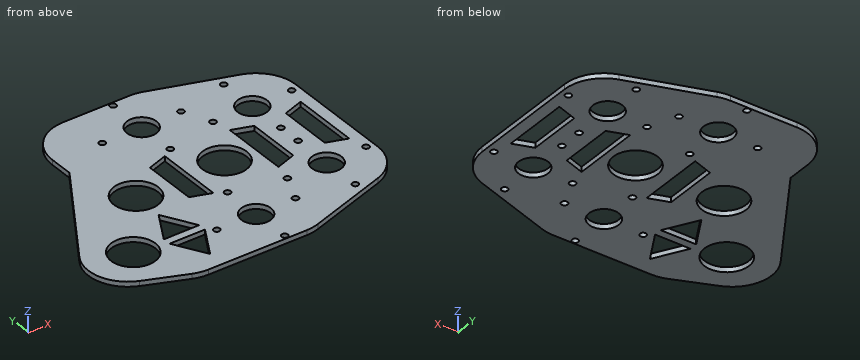
```python
from build123d import *

# Parameters (mm, degrees)
SKETCH1_R           = 14.2875
SKETCH1_R_2         = 9.525
BASE_FLANGE1_DEPTH  = 3.175
SKETCH2_R           = 2.032
CUT_EXTRUDE1_DEPTH  = 3.175
BREAK_CORNER1_START = -3.175
BREAK_CORNER1_DEPTH = 3.175
CUT_EXTRUDE2_DEPTH  = 3.175


# Read off the part's stored shape, not the designer's step: Break-Corner1
# Sheet-metal steps are written as plain solids
with BuildPart() as part:
    # Sketch1 → Base-Flange1 (new body)
    with BuildSketch(Plane.XY):
        Polygon((-72.39, 38.1), (-72.39, 78.74), (0, 78.74), (72.39, 54.946557626), (72.39, -54.946557626), (0, -78.74), (-72.39, -78.74), (-131.261342758, -54.940525177), align=None)
        Circle(SKETCH1_R, mode=Mode.SUBTRACT)
        with Locations((-16.51, 50.800692145)):
            Circle(SKETCH1_R_2, mode=Mode.SUBTRACT)
        with Locations(Location((-16.51, -50.800692145, 0), (0, 0, 180))):
            Circle(SKETCH1_R_2, mode=Mode.SUBTRACT)
        with Locations((-57.15, 0)):
            Circle(SKETCH1_R, mode=Mode.SUBTRACT)
        with Locations((-89.654815243, -42.291755533)):
            Circle(SKETCH1_R, mode=Mode.SUBTRACT)
        with Locations((41.987736572, 33.02)):
            Circle(SKETCH1_R_2, mode=Mode.SUBTRACT)
        with Locations((41.987736572, -33.02)):
            Circle(SKETCH1_R_2, mode=Mode.SUBTRACT)
    extrude(amount=-BASE_FLANGE1_DEPTH)

    # Sketch2 → Cut-Extrude1 (cut)
    with BuildSketch(Plane.XY):
        with Locations((-16.51, 76.200692145)):
            Circle(SKETCH2_R)
        with Locations((8.89, 50.800692145)):
            Circle(SKETCH2_R)
        with Locations(Location((-16.51, 25.400692145, 0), (0, 0, 180))):
            Circle(SKETCH2_R)
        with Locations(Location((-41.91, 50.800692145, 0), (0, 0, 180))):
            Circle(SKETCH2_R)
        with Locations((-41.91, -50.800692145)):
            Circle(SKETCH2_R)
        with Locations(Location((-16.51, -76.200692145, 0), (0, 0, 180))):
            Circle(SKETCH2_R)
        with Locations(Location((8.89, -50.800692145, 0), (0, 0, 180))):
            Circle(SKETCH2_R)
        with Locations((-16.51, -25.400692145)):
            Circle(SKETCH2_R)
        with Locations((41.987736572, 58.42)):
            Circle(SKETCH2_R)
        with Locations(Location((41.987736572, 7.62, 0), (0, 0, 180))):
            Circle(SKETCH2_R)
        with Locations((16.587736572, 33.02)):
            Circle(SKETCH2_R)
        with Locations(Location((67.387736572, 33.02, 0), (0, 0, 180))):
            Circle(SKETCH2_R)
        with Locations((41.987736572, -7.62)):
            Circle(SKETCH2_R)
        with Locations((67.387736572, -33.02)):
            Circle(SKETCH2_R)
        with Locations(Location((41.987736572, -58.42, 0), (0, 0, 180))):
            Circle(SKETCH2_R)
        with Locations(Location((16.587736572, -33.02, 0), (0, 0, 180))):
            Circle(SKETCH2_R)
    extrude(amount=-CUT_EXTRUDE1_DEPTH, mode=Mode.SUBTRACT)

    # Break-Corner1 outline → Break-Corner1 (cut)
    with BuildSketch(Plane.XY.offset(BREAK_CORNER1_START)):
        with BuildLine():
            ThreePointArc((-72.39, 53.34), (-64.950512242, 71.300512242), (-46.99, 78.74))
            Line((-46.99, 78.74), (-72.39, 78.74))
            Line((-72.39, 78.74), (-72.39, 53.34))
        make_face()
        with BuildLine():
            Line((0, 78.74), (-4.067255107, 78.74))
            ThreePointArc((-4.067255107, 78.74), (-0.051162479, 78.420490426), (3.863892351, 77.47))
            Line((3.863892351, 77.47), (0, 78.74))
        make_face()
        with BuildLine():
            ThreePointArc((-103.041642579, -66.34869106), (-117.701544329, -50.578489915), (-114.985920109, -29.218776702))
            Line((-114.985920109, -29.218776702), (-131.261342758, -54.940525177))
            Line((-131.261342758, -54.940525177), (-103.041642579, -66.34869106))
        make_face()
        with BuildLine():
            Line((72.39, 54.946557626), (54.921147458, 60.688291792))
            ThreePointArc((54.921147458, 60.688291792), (67.564391187, 51.453070316), (72.39, 36.558291792))
            Line((72.39, 36.558291792), (72.39, 54.946557626))
        make_face()
        with BuildLine():
            ThreePointArc((-67.450063518, -78.74), (-72.299143718, -78.27283821), (-76.969853447, -76.888537103))
            Line((-76.969853447, -76.888537103), (-72.39, -78.74))
            Line((-72.39, -78.74), (-67.450063518, -78.74))
        make_face()
        with BuildLine():
            Line((72.39, -54.946557626), (72.39, -36.558291792))
            ThreePointArc((72.39, -36.558291792), (67.564391187, -51.453070316), (54.921147458, -60.688291792))
            Line((54.921147458, -60.688291792), (72.39, -54.946557626))
        make_face()
        with BuildLine():
            ThreePointArc((3.863892351, -77.47), (-0.051162479, -78.420490426), (-4.067255107, -78.74))
            Line((-4.067255107, -78.74), (0, -78.74))
            Line((0, -78.74), (3.863892351, -77.47))
        make_face()
    extrude(amount=BREAK_CORNER1_DEPTH, mode=Mode.SUBTRACT)

    # Sketch3 → Cut-Extrude2 (cut)
    with BuildSketch(Plane.XY):
        Polygon((64.847736572, 21.59), (64.847736572, -21.59), (52.147736572, -17.272), (52.147736572, 17.272), align=None)
        Polygon((19.127736572, 21.59), (19.127736572, -21.59), (31.827736572, -17.272), (31.827736572, 17.272), align=None)
        Polygon((-35.56, -17.272), (-22.86, -21.59), (-22.86, 21.59), (-35.56, 17.272), align=None)
        Polygon((-58.214986183, -67.274834659), (-69.644986183, -46.954834659), (-46.784986183, -46.954834659), align=None)
        Polygon((-69.644986183, -41.874834659), (-58.214986183, -21.554834659), (-46.784986183, -41.874834659), align=None)
    extrude(amount=-CUT_EXTRUDE2_DEPTH, mode=Mode.SUBTRACT)


solid = part.part
```
Here's how the part is built. I have some questions about the finished solid (model axes, mm). Coordinates: 2 decimals unless noted, no trailing zeros. Order: outer loops, then holes, each group sorted by start corner. A loop starts at its lowest first (then second) coordinate and runs counter-clockwise, first axis right, second up. Notation, with made-up numbers: (22, -6) - (76, -6) arc R34 ccw to (76, 27) - close; hole circle Ø2 at (5.5, 8). An arc over 180 degrees is marked (long way). One line per question, with ' | ' between items.
(1) Suppose I cut it at D-D on y = -33.02. List the corners of the cut face in (x, z) for me (3 decimals), and give its area (3 significant figures).
Report:
outline: (-116.963, -3.175) - (-100.525, -3.175) - (-100.525, 0) - (-116.963, 0) - close; (-78.784, -3.175) - (-64.664, -3.175) - (-64.664, 0) - (-78.784, 0) - close; (-51.766, -3.175) - (14.556, -3.175) - (14.556, 0) - (-51.766, 0) - close; (18.62, -3.175) - (32.463, -3.175) - (32.463, 0) - (18.62, 0) - close; (51.513, -3.175) - (65.356, -3.175) - (65.356, 0) - (51.513, 0) - close; (69.42, -3.175) - (72.39, -3.175) - (72.39, 0) - (69.42, 0) - close | area: 405 mm2
(2) Will this pin go through, and if not, where does the flat tip stop? pin 1 (5 mm diameter, centred on x = -6.5, y = -12, fed in from +Z).
Report:
pin 1: stops at z = 0
(3) Suppose I cut it at B-B on y = 0. List the corners of the cut face in (x, z) for me (1 decimal).
Report:
outline: (-96.5, -3.2) - (-71.4, -3.2) - (-71.4, 0) - (-96.5, 0) - close; (-42.9, -3.2) - (-35.6, -3.2) - (-35.6, 0) - (-42.9, 0) - close; (-22.9, -3.2) - (-14.3, -3.2) - (-14.3, 0) - (-22.9, 0) - close; (14.3, -3.2) - (19.1, -3.2) - (19.1, 0) - (14.3, 0) - close; (31.8, -3.2) - (52.1, -3.2) - (52.1, 0) - (31.8, 0) - close; (64.8, -3.2) - (72.4, -3.2) - (72.4, 0) - (64.8, 0) - close
(4) Suppose I cut it at A-A on x = -16.51. List the corners of the cut face in (y, z) for me (3 decimals), and give its area (3 significant figures).
Report:
outline: (-78.74, -3.175) - (-78.233, -3.175) - (-78.233, 0) - (-78.74, 0) - close; (-74.169, -3.175) - (-60.326, -3.175) - (-60.326, 0) - (-74.169, 0) - close; (-41.276, -3.175) - (-27.433, -3.175) - (-27.433, 0) - (-41.276, 0) - close; (-23.369, -3.175) - (23.369, -3.175) - (23.369, 0) - (-23.369, 0) - close; (27.433, -3.175) - (41.276, -3.175) - (41.276, 0) - (27.433, 0) - close; (60.326, -3.175) - (74.169, -3.175) - (74.169, 0) - (60.326, 0) - close; (78.233, -3.175) - (78.74, -3.175) - (78.74, 0) - (78.233, 0) - close | area: 327 mm2
(5) Suppose I cut it at C-C on x = -98.5. List the corners of the cut face in (y, z) for me (3 decimals).
Report:
outline: (-68.185, -3.175) - (-53.512, -3.175) - (-53.512, 0) - (-68.185, 0) - close; (-31.071, -3.175) - (-3.164, -3.175) - (-3.164, 0) - (-31.071, 0) - close
(6) If I drill on L1, parallel to Y at x = -41.91, z = -1.8; L2, parallel to X at y = -50.5, z = -0.9; L3, parallel to X at y = -48.5, z = -1.75, over which ranges is the centre line in solid material (lowest first)?
Report:
L1: y = -78.74 to -52.83, -48.77 to 48.77, 52.83 to 78.74 | L2: x = -117.73 to -101.35, -77.96 to -67.65, -48.78 to -43.92, -39.9 to -26.03, -6.99 to 6.88, 10.9 to 68.22 | L3: x = -118.27 to -102.52, -76.79 to -68.78, -47.65 to -25.75, -7.27 to 69.41
